from build123d import *

# Parameters (mm, degrees)
F0_W     = 1524
F0_H     = 584.2
F1_DEPTH = 76.2
F5_DEPTH = 25.4


with BuildPart() as f1:
    # F0 (on Top) → F1 (new body)
    with BuildSketch(Plane.XY):
        Rectangle(F0_W, F0_H)
    extrude(amount=F1_DEPTH)

    # F4 (on offset) → F5 (join)
    with BuildSketch(Plane.XZ.offset(254)):
        Polygon((-644.339591, -25.4), (-695.333638, -25.4), (-762, -787.4), (-711.005952, -787.4), (-697.67268, -635), (-695.450468, -609.6), align=None)
        Polygon((762, -787.4), (695.333638, -25.4), (644.339591, -25.4), (695.450468, -609.6), (697.67268, -635), (711.005952, -787.4), align=None)
        Polygon((693.111426, 0), (-693.111426, 0), (-695.333638, -25.4), (-644.339591, -25.4), (644.339591, -25.4), (695.333638, -25.4), align=None)
        Polygon((695.450468, -609.6), (-695.450468, -609.6), (-697.67268, -635), (697.67268, -635), align=None)
    extrude(amount=F5_DEPTH)

    # F6: F1 across plane


with BuildPart() as f1_1:
    add(f1.part)
    add(f1.part.mirror(Plane.XZ))


solid = f1_1.part
Verification items for the finished model (mm, model axes). A direction names the side the tool comes from. Give positions to 0.01 mm unless a question says otherwise; leave off trailing zeros. Order: outer loops, then holes, each group sorted by start corner. A loop starts at its lowest first (then second) coordinate and runs counter-clockwise, first axis right, second up. Notation, with made-up numbers: M 47,-32 L 87,-32 A20 cw 87,-6 Z; hole C 28,-30 d11. An arc over 180 degrees is marked long. Answer as a JSON object with one key per item and string values. Group by question number.
1) Scan lines: line 1 along Y through (x, z) = (-206, -24); line 2 along Z through (x, y) = (-166.5, -208). Record each from-to range of solid material in increasing order. Write a range as [from, to].
2) Depth check by flat-ended pin: pin 1 Ø20.5 at (x, y) = (-151.5, 263) entering from -Z; pin 2 Ø10 at (x, y) = (404, 164.5) entering from -Z. Enter the tip coordinate at first touch or a pass-through.
3) Cross-section at A-A (x = 620). Enter the section's corners in (y, z).
4) Mould release check, pull along Y, two halves, no side actions. Record for faces 1 (the face through (-4, 279.4, -625)), 2 (the face through (-4, -254, -625)), 3 (the face through (-4, -279.4, -625)), 4 (the face through (-670.253, -266.522, -321.589)): released by +Y, released by -Y, zero draft, split by the parting line, or undercut.
5) Cross-section at B-B (z = -307). Enter the section's corners in (x, y), then the cut area to 3 significant figures.
6) Cross-section at C-C (y = -212.5). Enter the section's corners in (x, z).
7) Access from +Z, -Z, +X, -X, +Y, -Y to the whole of each face (thin tool, end or side, straight path). Record for faces 5 (the face through (-762, -4, 38)), 6 (the face through (-4, 254, -625)), 7 (the face through (669.537, 266.522, -313.411)).
Result sheet:
{
 "1": {"line 1": "y = [-279.4, -254], [254, 279.4]", "line 2": "z = [0, 76.2]"},
 "2": {"pin 1": "stops at z = -635", "pin 2": "stops at z = 0"},
 "3": {"outline": "M -292.1,0 L -279.4,0 L -279.4,-25.4 L -254,-25.4 L -254,0 L 254,0 L 254,-25.4 L 279.4,-25.4 L 279.4,0 L 292.1,0 L 292.1,76.2 L -292.1,76.2 Z; M -279.4,-635 L -254,-635 L -254,-609.6 L -279.4,-609.6 Z; M 254,-635 L 279.4,-635 L 279.4,-609.6 L 254,-609.6 Z"},
 "4": {"face 1": "released by +Y", "face 2": "undercut", "face 3": "released by -Y", "face 4": "zero draft"},
 "5": {"outline": "M -719.97,-279.4 L -668.98,-279.4 L -668.98,-254 L -719.97,-254 Z; M -719.97,254 L -668.98,254 L -668.98,279.4 L -719.97,279.4 Z; M 668.98,-279.4 L 719.97,-279.4 L 719.97,-254 L 668.98,-254 Z; M 668.98,254 L 719.97,254 L 719.97,279.4 L 668.98,279.4 Z", "area": "5,180 mm2"},
 "6": {"outline": "M -762,0 L 762,0 L 762,76.2 L -762,76.2 Z"},
 "7": {"face 5": "+Z, -Z, -X, +Y, -Y", "face 6": "-Z, +X, -X", "face 7": "+Y, -Y"}
}
